from build123d import *

# Parameters (mm, degrees)
F0_R     = 9.0613386753
F0_W     = 16.764
F0_H     = 5.08
F0_W_2   = 16.7640029008
F1_DEPTH = 25.4
F2_W     = 13.3351978731
F2_H     = 6.8151620217
F3_DEPTH = 25.4
F4_R     = 2.3131415356
F5_DEPTH = 127


with BuildPart() as f1:
    # F0 (on Top) → F1 (new body)
    with BuildSketch(Plane.XY):
        with BuildLine():
            ThreePointArc((-19.3765729799, -9.5403834533), (-16.4600808117, -5.1610380229), (-15.4362256016, 0))
            ThreePointArc((-15.4362256016, 0), (-16.4600808117, 5.1610380229), (-19.3765729799, 9.5403834533))
            Line((-19.3765729799, 9.5403834533), (-19.3765729799, -9.5403834533))
        make_face()
        with BuildLine():
            ThreePointArc((-19.3765729799, 9.5403834533), (-16.4600808117, 5.1610380229), (-15.4362256016, 0))
            ThreePointArc((-15.4362256016, 0), (-16.4600808117, -5.1610380229), (-19.3765729799, -9.5403834533))
            Line((-19.3765729799, -9.5403834533), (-19.3765729799, -19.4854322))
            Line((-19.3765729799, -19.4854322), (-11.7565729799, -19.4854322))
            Line((-11.7565729799, -19.4854322), (-11.7565729799, -14.4054322))
            Line((-11.7565729799, -14.4054322), (-11.7565729799, 14.4054288318))
            Line((-11.7565729799, 14.4054288318), (-11.7565729799, 19.4854288318))
            Line((-11.7565729799, 19.4854288318), (-19.3765729799, 19.4854288318))
            Line((-19.3765729799, 19.4854288318), (-19.3765729799, 9.5403834533))
        make_face()
        with BuildLine():
            Line((-19.3765729799, -9.5403834533), (-19.3765729799, 9.5403834533))
            ThreePointArc((-19.3765729799, 9.5403834533), (-42.4757842164, 0), (-19.3765729799, -9.5403834533))
        make_face()
        with Locations((-28.956004909, 0)):
            Circle(F0_R, mode=Mode.SUBTRACT)
        with Locations((-3.3745729799, 16.9454288318)):
            Rectangle(F0_W, F0_H)
        with Locations((-3.3745715295, -16.9454322)):
            Rectangle(F0_W_2, F0_H)
    extrude(amount=F1_DEPTH)

    # F2 (on face) → F3 (cut)
    with BuildSketch(Plane.XY.offset(25.4)):
        with Locations((-38.0173435843, 0)):
            Rectangle(F2_W, F2_H)
    extrude(amount=-F3_DEPTH, mode=Mode.SUBTRACT)

    # F4 (on Front) → F5 (cut, symmetric)
    with BuildSketch(Plane.XZ):
        with Locations((-38.4375117719, 14.0392342582)):
            Circle(F4_R)
    extrude(amount=F5_DEPTH, both=True, mode=Mode.SUBTRACT)


solid = f1.part
Work out the finished part from the listing and answer in its coordinate system (mm). A direction names the side the tool comes from. Round coordinates to 2 decimals unless told otherwise and drop trailing zeros. Loops run counter-clockwise (first coordinate to the right, second up) from the corner with the lowest first, then second, coordinate; pieces in that order, holes last. Notation, with made-up numbers: (59.5, 30.25) - (82.5, 30.25) arc R26 cw to (82.5, 47.25) - close; hole circle Ø7 at (-18.5, 39.5). An arc over 180 degrees is marked (long way). One line per item, written item: value.
Q1. For faces 5 (the flat face through (-3, 14.405, 13)), 6 (the flat face through (-41, 3.408, 13)), 7 (the flat face through (-19.377, 15, 13)), determine the directions among +Z, -Z, +X, -X, +Y, -Y from which every point of the face is accessible in a straight line to the end or side of a thin tool.
Check values:
face 5: +Z, -Z, +X
face 6: +Z, -Z, -X
face 7: +Z, -Z, +Y
Q2. The mould has two halves that part along Y. Classify faces 1 (the flat face through (-7, 19.485, 13)), 2 (the flat face through (-41, -3.408, 13)), 3 (the flat face through (-19, 0, 25.4)), 4 (the flat face through (-11.757, 0, 13)): +Y half, -Y half, draft (parallel to the pull), parting line (faces both ways), or undercut.
Check values:
face 1: +Y half
face 2: undercut
face 3: draft
face 4: undercut
Q3. Straight lines are drawn through the part: probe 1 along Y at (x, z) = (-9.5, 10.5); probe 2 along Y at (x, z) = (-28.5, 11); probe 3 along X at (y, z) = (14, 11.75). For each, find the intervals that lie inside material, in ascending order.
Check values:
probe 1: -19.49 to -14.41, 14.41 to 19.49
probe 2: -13.51 to -9.05, 9.05 to 13.51
probe 3: -19.38 to -11.76
Q4. Each of these flat-tipped pins is pushed along its axis until it touches: pin 1 Ø3 at (y, z) = (12.5, 10.5) entering from -X; pin 2 Ø7.5 at (x, z) = (-38.44, 14.04) entering from -Y; pin 3 Ø4 at (y, z) = (10.5, 4.5) entering from -X; pin 4 Ø14.5 at (x, y) = (-28.96, 0) entering from -Z. Where does it stop, or does it pass through?
Check values:
pin 1: x = -36.82
pin 2: y = -12.24
pin 3: x = -39.47
pin 4: through
Q5. Find section A-A on x = -9. Give the vertices of the cut face in (y, z), and give its area (3 significant figures).
Check values:
outline: (-19.49, 0) - (-14.41, 0) - (-14.41, 25.4) - (-19.49, 25.4) - close; (14.41, 0) - (19.49, 0) - (19.49, 25.4) - (14.41, 25.4) - close
area: 258 mm2
Q6. Find section D-D on x = -32. Give the vertices of the cut face in (y, z), and give its area (3 significant figures).
Check values:
outline: (-13.17, 0) - (-8.53, 0) - (-8.53, 25.4) - (-13.17, 25.4) - close; (8.53, 0) - (13.17, 0) - (13.17, 25.4) - (8.53, 25.4) - close
area: 236 mm2
Q7. Find section B-B on y = -7.5. Give the vertices of the cut face in (x, z).
Check values:
outline: (-40.2, 0) - (-34.04, 0) - (-34.04, 25.4) - (-40.2, 25.4) - (-40.2, 15.53) arc R2.31 cw (long way) to (-40.2, 12.55) - close; (-23.87, 0) - (-11.76, 0) - (-11.76, 25.4) - (-23.87, 25.4) - close
Q8. Find section C-C on z = 24. Give the vertices of the cut face in (x, y).
Check values:
outline: (-42.04, -3.41) arc R13.52 ccw to (-19.38, -9.54) - (-19.38, -19.49) - (5.01, -19.49) - (5.01, -14.41) - (-11.76, -14.41) - (-11.76, 14.41) - (5.01, 14.41) - (5.01, 19.49) - (-19.38, 19.49) - (-19.38, 9.54) arc R13.52 ccw to (-42.04, 3.41) - (-37.35, 3.41) arc R9.06 cw (long way) to (-37.35, -3.41) - close
